from build123d import *

# Parameters (mm, degrees)
F0_R     = 56
F1_DEPTH = 23
F2_R     = 46
F3_DEPTH = 3
F5_ANGLE = -180


with BuildPart() as f1:
    # F0 (on Top) → F1 (new body)
    with BuildSketch(Plane.XY):
        Circle(F0_R)
    extrude(amount=-F1_DEPTH)

    # F2 (on face) → F3 (cut)
    with BuildSketch(Plane.XY):
        Circle(F2_R)
    extrude(amount=-F3_DEPTH, mode=Mode.SUBTRACT)

    # F4 (on face) → F5 (revolve, cut)
    with BuildSketch(Plane.XY.offset(-3)):
        with BuildLine():
            Line((0, -40), (0, 40))
            ThreePointArc((0, 40), (-40, 0), (0, -40))
        make_face()
    revolve(axis=Axis((0, 0, -3), (0, 1, 0)), revolution_arc=F5_ANGLE, mode=Mode.SUBTRACT)


solid = f1.part
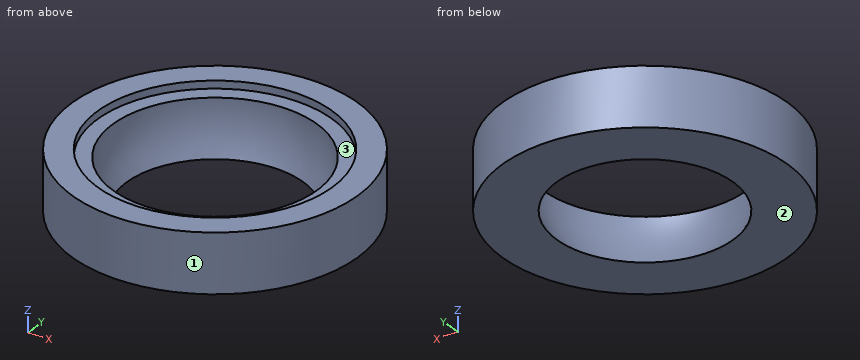
Can you work these out from the model? Positions are in its coordinate system, mm. Face numbers are marked on the shaded views. Give positions to 0.01 mm unless a question says otherwise; leave off trailing zeros. Write each loop counter-clockwise with the first axis right and the second up, starting at its lowest first coordinate (ties: lowest second). Pieces come first, ordered by that corner, then holes. Notation, with made-up numbers: (15.25, 49) -> (36.25, 49) arc R23 ccw to (36.25, 81) -> close; hole circle Ø1 at (2, 58.5). An arc over 180 degrees is marked (long way). Answer as a JSON object with one key per item and string values. Group by question number.
Item 1: Suppose I cut it at B-B (x = 4). Please give me the cut outline in (y, z).
Item 2: I'm going to push flat-ended pins straight in: P1, Ø2, axis at y = 10.5, z = -16, coming from the -X side; P2, Ø6, axis at x = 45, y = -2.5, coming from the +Z side; P3, Ø4, axis at x = 9.5, z = -4.5, coming from the +Y side; P4, Ø1, axis at x = -31.5, z = -12.5, coming from the +Y side. Where does each tip first touch, or does it pass through?
Item 3: Suppose I cut it at C-C (z = -17.75). Please give me the cut outline in (x, y).
Item 4: Suppose I cut it at A-A (y = -32.5). Please give me the cut outline in (x, z), plus the area to 3 significant figures.
Item 5: Suppose I cut it at D-D (y = 35). Please give me the cut outline in (x, z), plus the area to 3 significant figures.
Item 6: Please list where these lines run through material, in increasing order: line 1 (Y direction, x = 0, z = -1); line 2 (Y direction, x = 5, z = -11.5); line 3 (Z direction, x = -35.5, y = -25.5). Write a range as [from, to].
Item 7: We'd pull the mould along Y, two halves only. Please class the marked faces 1, 2 and 3: +Y half, -Y half, draft (parallel to the pull), parting line (faces both ways), or undercut.
Findings:
{
 "1": {"outline": "(-55.86, -23) -> (-34.41, -23) arc R39.8 cw to (-39.8, -3) -> (-45.83, -3) -> (-45.83, 0) -> (-55.86, 0) -> close; (34.41, -23) -> (55.86, -23) -> (55.86, 0) -> (45.83, 0) -> (45.83, -3) -> (39.8, -3) arc R39.8 cw to start"},
 "2": {"P1": "stops at x = -55.19", "P2": "stops at z = 0", "P3": "stops at y = 55.5", "P4": "stops at y = 46.64"},
 "3": {"outline": "circle Ø112 at (0, 0); hole circle Ø74.36 at (0, 0)"},
 "4": {"outline": "(-45.6, -23) -> (-11.99, -23) arc R23.32 cw to (-23.32, -3) -> (-32.55, -3) -> (-32.55, 0) -> (-45.6, 0) -> close; (11.99, -23) -> (45.6, -23) -> (45.6, 0) -> (32.55, 0) -> (32.55, -3) -> (23.32, -3) arc R23.32 cw to start", "area": "1,100 mm²"},
 "5": {"outline": "(-43.71, -23) -> (43.71, -23) -> (43.71, 0) -> (29.85, 0) -> (29.85, -3) -> (19.36, -3) arc R19.36 cw to (-19.36, -3) -> (-29.85, -3) -> (-29.85, 0) -> (-43.71, 0) -> close", "area": "1,240 mm²"},
 "6": {"line 1": "y = [-56, -46], [46, 56]", "line 2": "y = [-55.78, -38.77], [38.77, 55.78]", "line 3": "z = [-23, -3]"},
 "7": {"face 1": "parting line", "face 2": "draft", "face 3": "undercut"}
}
